from build123d import *

# Parameters (mm, degrees)
SKETCH1_R           = 20.6
BOSS_EXTRUDE1_DEPTH = 2
SKETCH2_R           = 5.15
CUT_EXTRUDE1_DEPTH  = 3
SKETCH3_R           = 6.5
CUT_EXTRUDE2_DEPTH  = 2
BOSS_EXTRUDE4_DEPTH = 22
FILLET2_R           = 6


with BuildPart() as part:
    # Sketch1 → Boss-Extrude1 (new body)
    with BuildSketch(Plane(origin=(0, 0, 0), x_dir=(1, 0, 0), z_dir=(0, 1, 0))):
        with Locations(Location((0, 0, 0), (0, 0, 270))):
            Circle(SKETCH1_R)
    extrude(amount=BOSS_EXTRUDE1_DEPTH)

    # Sketch2 → Cut-Extrude1 (cut)
    with BuildSketch(Plane(origin=(0, 2, 0), x_dir=(1, 0, 0), z_dir=(0, 1, 0))):
        with Locations(Location((0, 0, 0), (0, 0, 270))):
            Circle(SKETCH2_R)
    extrude(amount=-CUT_EXTRUDE1_DEPTH, mode=Mode.SUBTRACT)

    # Sketch3 → Cut-Extrude2 (cut)
    with BuildSketch(Plane(origin=(0, 2, 0), x_dir=(1, 0, 0), z_dir=(0, 1, 0))):
        with Locations(Location((0, 13, 0), (0, 0, 270))):
            Circle(SKETCH3_R)
    extrude(amount=-CUT_EXTRUDE2_DEPTH, mode=Mode.SUBTRACT)

    # Sketch4 → Boss-Extrude4 (add)
    with BuildSketch(Plane(origin=(0, 2, 0), x_dir=(1, 0, 0), z_dir=(0, 1, 0))):
        with BuildLine():
            Line((-16.743954133, 12), (-3.5, 5.5))
            Line((-3.5, 5.5), (3.5, 5.5))
            Line((3.5, 5.5), (16.743954133, 12))
            ThreePointArc((16.743954133, 12), (13.279606143, 15.748398671), (9, 18.529975715))
            ThreePointArc((9, 18.529975715), (0, 6.042759079), (-9, 18.529975715))
            ThreePointArc((-9, 18.529975715), (-13.279606143, 15.748398671), (-16.743954133, 12))
        make_face()
    extrude(amount=BOSS_EXTRUDE4_DEPTH)

    # Fillet2
    # the kernel refuses this fillet: 6 mm, written as the material it takes off along each edge
    with BuildSketch(Plane(origin=(16.743954133, 2, -12), x_dir=(-0.7761796310564387, 0, -0.6305118399626535), z_dir=(0, 1, 0))) as fillet2_piece_1:
        with BuildLine():
            CenterArc((9.278744028, 5.78779133), FILLET2_R, 155.229237023, 130.054584679)
            Line((3.830795632, 8.301724161), (0, 0))
            ThreePointArc((0, 0), (5.430174062, -0.728583099), (10.860348123, 0))
        make_face()
    extrude(amount=49.150870308, mode=Mode.SUBTRACT)
    with BuildSketch(Plane(origin=(-16.743954133, 2, -12), x_dir=(0.7761796310564387, 0, -0.6305118399626534), z_dir=(0, 1, 0))) as fillet2_piece_2:
        with BuildLine():
            CenterArc((9.278744028, -5.78779133), FILLET2_R, 74.716178298, 130.054584679)
            Line((3.830795632, -8.301724161), (0, 0))
            ThreePointArc((0, 0), (5.430174062, 0.728583099), (10.860348123, 0))
        make_face()
    extrude(amount=49.150870308, mode=Mode.SUBTRACT)


solid = part.part
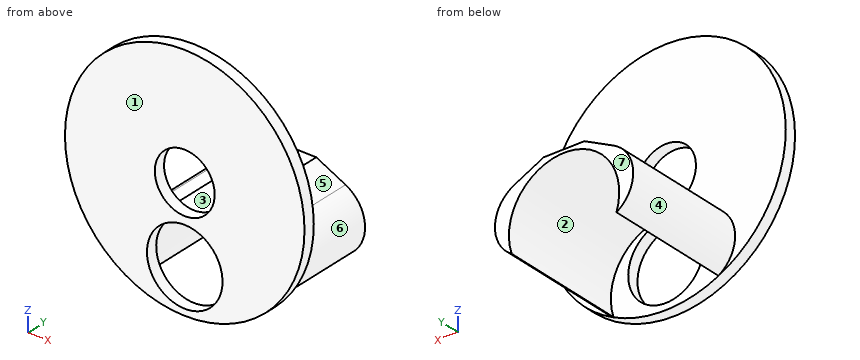
Verification items for the finished model (mm, model axes). Face numbers are marked on the shaded views. A direction names the side the tool comes from. Give positions to 0.01 mm unless a question says otherwise; leave off trailing zeros. Loops run counter-clockwise (first coordinate to the right, second up) from the corner with the lowest first, then second, coordinate; pieces in that order, holes last.
1) Sectioned sample at D-D, the plane z = 7. Enter the section's corners in (x, y).
2) Depth check by flat-ended pin: pin 1 Ø1.5 at (x, z) = (-15.5, 8.5) entering from +Y; pin 2 Ø6 at (x, y) = (-9.5, 17.5) entering from +Z; pin 3 Ø4 at (y, z) = (5.5, -6.5) entering from -X. Enter the tip coordinate at first touch or a pass-through.
3) Thickness scan on line 1 along X through (y, z) = (0.5, 0); line 2 along Z through (x, y) = (-2, 1.5); line 3 along Y through (x, z) = (-8.5, 18). Record the ranges inside material, lowest first.
4) Sectioned sample at B-B, the plane z = 0. Enter the section's corners in (x, y).
5) Set-up check for the marked faces 4, 5, 6 and 7: record each of +Z, -Z, +X, -X, +Y, -Y from which the full face is reachable in a straight line by a thin tool's end or side.
6) Sectioned sample at A-A, the plane x = 0. Enter the section's corners in (y, z).
7) Draft check along Z on the marked faces 1, 2 and 3. Enter one of: pulls with the +Z half, pulls with the -Z half, needs draft (parallel to the pull), parting line crosses it, or undercut.
8) Sectioned sample at C-C, the plane z = -13. Enter the section's corners in (x, y), then the cut area to 3 significant figures.
Answers:
1. outline: (-19.37, 0) - (19.37, 0) - (19.37, 2) - (-19.37, 2) - close
2. pin 1: stops at y = 2
2. pin 2: stops at z = -6.97
2. pin 3: stops at x = -9.41
3. line 1: x = -20.6 to -5.15, 5.15 to 20.6
3. line 2: z = -20.5 to -19.18, -6.82 to -4.75, 4.75 to 20.5
3. line 3: y = 0 to 2
4. outline: (-20.6, 0) - (-5.15, 0) - (-5.15, 2) - (-20.6, 2) - close; (5.15, 0) - (20.6, 0) - (20.6, 2) - (5.15, 2) - close
5. face 4: -X, +Y
5. face 5: +Z, +X, +Y
5. face 6: +X, +Y
5. face 7: +Z, -Z, +X, -X, +Y
6. outline: (0, -20.6) - (2, -20.6) - (2, -19.5) - (0, -19.5) - close; (0, -6.5) - (2, -6.5) - (2, -6.04) - (24, -6.04) - (24, -5.5) - (2, -5.5) - (2, -5.15) - (0, -5.15) - close; (0, 5.15) - (2, 5.15) - (2, 20.6) - (0, 20.6) - close
7. face 1: needs draft
7. face 2: undercut
7. face 3: pulls with the +Z half
8. outline: (-15.98, 0) - (-6.5, 0) - (-6.5, 2) - (-9.14, 2) - (-9.14, 24) - (-11.88, 24) - (-11.88, 2) - (-15.98, 2) - close; (6.5, 0) - (15.98, 0) - (15.98, 2) - (11.88, 2) - (11.88, 24) - (9.14, 24) - (9.14, 2) - (6.5, 2) - close
8. area: 158 mm2
